from build123d import *

# Parameters (mm, degrees)
BOSS_EXTRUDE1_DEPTH      = 50
BOSS_EXTRUDE1_DEPTH_BACK = 50
SKETCH2_W                = 200
SKETCH2_H                = 130
SKETCH4_R                = 5
BOSS_EXTRUDE2_DEPTH      = 20
CUT_EXTRUDE1_DEPTH       = 142
SKETCH8_W                = 200.147061324
SKETCH8_H                = 101.72915409
CUT_EXTRUDE2_DEPTH       = 142


with BuildPart() as part:
    # Sketch2 → Boss-Extrude1 (new, two sides: drawn at the far end of the back side and taken through both)
    with BuildSketch(Plane(origin=(0, 0, 0), x_dir=(1, 0, 0), z_dir=(0, 1, 0)).offset(-BOSS_EXTRUDE1_DEPTH_BACK)):
        Rectangle(SKETCH2_W, SKETCH2_H)
    extrude(amount=BOSS_EXTRUDE1_DEPTH + BOSS_EXTRUDE1_DEPTH_BACK)

    # Sketch4 → Boss-Extrude2 (add)
    with BuildSketch(Plane.XY.offset(65)):
        Circle(SKETCH4_R)
    extrude(amount=BOSS_EXTRUDE2_DEPTH)

    # Sketch6 → Revolve1 (revolve)
    with BuildSketch(Plane.ZY.offset(100)):
        with BuildLine():
            Line((-35, -5), (-35, 45))
            ThreePointArc((-35, 45), (-10, 20), (-35, -5))
        make_face()
    revolve1 = revolve(axis=Axis((-100, -5, -35), (0, 1, 0)))

    # Mirror1: Revolve1 across plane
    add(revolve1.mirror(Plane(origin=(0, 0, 0), x_dir=(0, 0, 1), z_dir=(1, 0, 0))))

    # Sketch7 → Cut-Extrude1 (cut)
    with BuildSketch(Plane(origin=(0, 0, -65), x_dir=(-1, 0, 0), z_dir=(0, 0, -1))):
        with BuildLine():
            ThreePointArc((-37.519288456, -50), (-68.867740428, -47.018454326), (-100, -42.285857823))
            Line((-100, -42.285857823), (-100, -50))
            Line((-100, -50), (-37.519288456, -50))
        make_face()
        with BuildLine():
            Line((100, -50), (100, -42.285857823))
            ThreePointArc((100, -42.285857823), (68.867740428, -47.018454326), (37.519288456, -50))
            Line((37.519288456, -50), (100, -50))
        make_face()
    extrude(amount=-CUT_EXTRUDE1_DEPTH, mode=Mode.SUBTRACT)

    # Sketch8 → Cut-Extrude2 (cut)
    with BuildSketch(Plane(origin=(0, 50, 0), x_dir=(1, 0, 0), z_dir=(0, 1, 0))):
        with Locations((0.073530662, -50.864577045)):
            Rectangle(SKETCH8_W, SKETCH8_H)
    extrude(amount=-CUT_EXTRUDE2_DEPTH, mode=Mode.SUBTRACT)


solid = part.part
Model file for the job. Use its own axes, mm. Give positions to 0.01 mm unless a question says otherwise; leave off trailing zeros. Write each loop counter-clockwise with the first axis right and the second up, starting at its lowest first coordinate (ties: lowest second). Pieces come first, ordered by that corner, then holes. Notation, with made-up numbers: (-35, -7) - (10, -7) arc R35 ccw to (10, 29) - close; hole circle Ø5 at (26.5, -8). An arc over 180 degrees is marked (long way). Answer as CSV lines item,"result".
1. Band-saw the part on A-A (z = -28). Write the cut outline in (x, y).
Responses:
outline,"(-100, -42.29) arc R562.03 ccw to (-37.52, -50) - (37.52, -50) arc R562.03 ccw to (100, -42.29) - (100, -4) arc R24 ccw to (100, 44) - (100, 50) - (-100, 50) - (-100, 44) arc R24 ccw to (-100, -4) - close"
2. Drill centre lines: L1, parallel to X at y = -20, z = -38; L2, parallel to Y at x = 106.5, z = -44.5; L3, parallel to X at y = 10, z = -17.5. Where is each one in solid material? Low to high. Write a range as [from, to].
Responses:
L1,"x = [-100, 100]"
L2,"y = [-2.19, 42.19]"
L3,"x = [-114.79, 114.79]"
3. Two-plate mould, pull along Y, no slides. Class faces 1 (the face through (-1, -50, -33)), 2 (the face through (-1, -1, -65)), 3 (the face through (-1, 50, -33)): +Y half, -Y half, draft (parallel to the pull), parting line (faces both ways), or undercut.
Responses:
face 1,"-Y half"
face 2,"draft"
face 3,"+Y half"
4. Band-saw the part on B-B (y = -23.5). Write the cut outline in (x, z), and give its area (3 significant figures).
Responses:
outline,"(-100, -65) - (100, -65) - (100, 0) - (-100, 0) - close"
area,"13,000 mm2"
5. Band-saw the part on C-C (z = -16). Write the cut outline in (x, y).
Responses:
outline,"(-100, -42.29) arc R562.03 ccw to (-37.52, -50) - (37.52, -50) arc R562.03 ccw to (100, -42.29) - (100, 3.75) arc R16.25 ccw to (100, 36.25) - (100, 50) - (-100, 50) - (-100, 36.25) arc R16.25 ccw to (-100, 3.75) - close"
6. Pin check, flat tips, straight feed: pin 1 (19.5 mm diameter, centred on y = -13, z = -48.5, fed in from -X); pin 2 (12 mm diameter, centred on y = 4.5, z = -37, fed in from -X); pin 3 (1.5 mm diameter, centred on x = -87, z = -53, fed in from -Y). Stop position of each tip, or through.
Responses:
pin 1,"stops at x = -100"
pin 2,"stops at x = -123.07"
pin 3,"stops at y = -44.6"
7. Band-saw the part on D-D (x = 83.5). Write the cut outline in (y, z), and give its area (3 significant figures).
Responses:
outline,"(-45.02, -65) - (50, -65) - (50, 0) - (-45.02, 0) - close"
area,"6,180 mm2"
